from build123d import *

# Parameters (mm, degrees)
SKETCH_1_R      = 2.5
SKETCH_1_R_2    = 0.5
EXTRUDE_1_DEPTH = 1


with BuildPart() as part:
    # 草图1 → 凸台-拉伸1 (new body)
    # profile 1 of 3: a face of its own
    with BuildSketch(Plane(origin=(0, 0, 0), x_dir=(1, 0, 0), z_dir=(0, 1, 0))):
        with BuildLine():
            Line((-21.398771617, -6.952882373), (-2.377641291, -0.772542486))
            ThreePointArc((-2.377641291, -0.772542486), (-2.469220851, -0.391086163), (-2.5, 0))
            Line((-2.5, 0), (-22.5, 0))
            ThreePointArc((-22.5, 0), (-22.222987663, -3.519775463), (-21.398771617, -6.952882373))
        make_face()
    # profile 2 of 3: a face of its own
    with BuildSketch(Plane(origin=(0, 0, 0), x_dir=(1, 0, 0), z_dir=(0, 1, 0))):
        with BuildLine():
            ThreePointArc((2.377641291, 0.772542486), (2.469220851, 0.391086163), (2.5, 0))
            Line((2.5, 0), (22.5, 0))
            ThreePointArc((22.5, 0), (22.222987663, 3.519775463), (21.398771617, 6.952882373))
            Line((21.398771617, 6.952882373), (2.377641291, 0.772542486))
        make_face()
    # profile 3 of 3: a face of its own
    with BuildSketch(Plane(origin=(0, 0, 0), x_dir=(1, 0, 0), z_dir=(0, 1, 0))):
        Circle(SKETCH_1_R)
        with Locations(Location((0, 0, 0), (0, 0, 270))):
            Circle(SKETCH_1_R_2, mode=Mode.SUBTRACT)
    extrude(amount=EXTRUDE_1_DEPTH)


solid = part.part
Geometry: final body of the model. Coordinates: model frame, mm. A direction names the side the tool comes from. Give positions to 0.01 mm unless a question says otherwise; leave off trailing zeros. Write each loop counter-clockwise with the first axis right and the second up, starting at its lowest first coordinate (ties: lowest second). Pieces come first, ordered by that corner, then holes. Notation, with made-up numbers: (-1.75, 22) - (20.25, 22) arc R16 cw to (20.25, 31) - close; hole circle Ø2 at (31.25, -28.5). An arc over 180 degrees is marked (long way). Return JSON: item names as keys, results as strings. Group by question number.
1) Section B-B on y = 0.2. Return the cut outline in (x, z).
2) Line query: line 1 (Z direction, x = -4.5, y = 0.25); line 2 (Z direction, x = -9, y = 0.2). Output: solid intervals per line, ascending.
3) Section D-D on z = 4.25. Return the cut outline in (x, y).
4) Section C-C on x = 0. Return the cut outline in (y, z), plus the area to 3 significant figures.
5) Section A-A on z = 1.75. Return the cut outline in (x, y), plus the area to 3 significant figures.
6) Set-up query: faces 4 (the flat face through (12, 0.5, -3.9)), 5 (the flat face through (-12, 0.5, 3.9)), 6 (the cylindrical face through (-0.488, 0.493, -0.108)), 7 (the flat face through (12.4, 0.5, 0)). Return all of +Z, -Z, +X, -X, +Y, -Y with unobstructed straight access to the full face (end or side cutting, diameter ignored); none if empty.
7) Mould query, pull axis X, two halves, no side actions, for faces 1 (the cylindrical face through (-22.23, 0.49, 3.47)), 2 (the flat face through (-12.4, 0.5, 0)), 3 (the cylindrical face through (0.342, 0.493, 2.476)). Classes: released by +X, released by -X, zero draft, split by the parting line, or undercut.
Filled in:
{
 "1": {"outline": "(-22.5, 0) - (-2.5, 0) arc R2.5 ccw to (2.38, -0.77) - (21.4, -6.95) arc R22.5 ccw to (22.5, 0) - (2.5, 0) arc R2.5 ccw to (-2.38, 0.77) - (-21.4, 6.95) arc R22.5 ccw to start; hole circle Ø1 at (0, 0)"},
 "2": {"line 1": "z = 0 to 1.46", "line 2": "z = 0 to 2.92"},
 "3": {"outline": "(-22.09, 0) - (-13.08, 0) - (-13.08, 1) - (-22.09, 1) - close"},
 "4": {"outline": "(0, -2.5) - (1, -2.5) - (1, -0.5) - (0, -0.5) - close; (0, 0.5) - (1, 0.5) - (1, 2.5) - (0, 2.5) - close", "area": "4.00 mm^2"},
 "5": {"outline": "(-22.43, 0) - (-5.39, 0) - (-5.39, 1) - (-22.43, 1) - close; (-1.79, 0) - (1.79, 0) - (1.79, 1) - (-1.79, 1) - close", "area": "20.6 mm^2"},
 "6": {"face 4": "-Z, +Y, -Y", "face 5": "+Z, +Y, -Y", "face 6": "+Y, -Y", "face 7": "+Z, +X, +Y, -Y"},
 "7": {"face 1": "released by -X", "face 2": "zero draft", "face 3": "undercut"}
}
